from build123d import *

# Parameters (mm, degrees)
MODEL_R                  = 1.8
RESSALTO_EXTRUS_O1_DEPTH = 6


with BuildPart() as part:
    # Model → Ressalto-extrusão1 (new body)
    with BuildSketch(Plane.XY):
        Polygon((36.676362522, 11.559126959), (43.318311298, 11.559126959), (48.38117681, 16.621992471), (46.093165841, 35.592208395), (45.494331575, 40.442304919), (44.330954819, 41.605681674), (35.830954819, 41.605681674), (34.69889139, 40.473618245), (31.60820441, 16.627285071), align=None)
        with Locations((40.079692562, 35.592208395)):
            Circle(MODEL_R, mode=Mode.SUBTRACT)
    extrude(amount=RESSALTO_EXTRUS_O1_DEPTH)


solid = part.part
Read the model definition and answer for the solid it produces. Units are mm, in the model's axes. Coordinates: 2 decimals unless noted, no trailing zeros. Loops run counter-clockwise (first coordinate to the right, second up) from the corner with the lowest first, then second, coordinate; pieces in that order, holes last. Notation, with made-up numbers: (-3.75, 15.5) -> (8.25, 15.5) arc R26 ccw to (8.25, 40.5) -> close; hole circle Ø7 at (-12.5, 20.25). An arc over 180 degrees is marked (long way). Answer in a Markdown table with one row per item.
Item 1: A cutting plane is placed at B-B on x = 41.5. Determine the outline of the cut face in (y, z).
Returned:
| item | result |
|---|---|
| outline | (11.56, 0) -> (34.49, 0) -> (34.49, 6) -> (11.56, 6) -> close; (36.7, 0) -> (41.61, 0) -> (41.61, 6) -> (36.7, 6) -> close |
Item 2: This flat-tipped pin is pushed along its axis until it touches: P1, Ø4.5, axis at x = 40.08, y = 35.59, coming from the -Z side. Where does it stop, or does it pass through?
Returned:
| item | result |
|---|---|
| P1 | stops at z = 0 |
Item 3: A cutting plane is placed at A-A on z = 4.7. Determine the outline of the cut face in (x, y), plus the area to 3 significant figures.
Returned:
| item | result |
|---|---|
| outline | (31.61, 16.63) -> (36.68, 11.56) -> (43.32, 11.56) -> (48.38, 16.62) -> (46.09, 35.59) -> (45.49, 40.44) -> (44.33, 41.61) -> (35.83, 41.61) -> (34.7, 40.47) -> close; hole circle Ø3.6 at (40.08, 35.59) |
| area | 389 mm^2 |
Item 4: For a pull along X with two mould halves and no side action, classify faces 1 (the flat face through (35.273, 41.048, 2.958)), 2 (the flat face through (40, 41.606, 3)), 3 (the flat face through (44.921, 41.016, 2.958)), 4 (the cylindrical face through (41.797, 36.133, 2.958)) as released by +X, released by -X, zero draft, split by the parting line, or undercut.
Returned:
| item | result |
|---|---|
| face 1 | released by -X |
| face 2 | zero draft |
| face 3 | released by +X |
| face 4 | undercut |
Item 5: A cutting plane is placed at D-D on x = 34. Determine the outline of the cut face in (y, z), plus the area to 3 significant figures.
Returned:
| item | result |
|---|---|
| outline | (14.24, 0) -> (35.08, 0) -> (35.08, 6) -> (14.24, 6) -> close |
| area | 125 mm^2 |
Item 6: Straight lines are drawn through the part: line 1 along Y through (x, z) = (40.25, 0.7); line 2 along Y through (x, z) = (40.5, 3.45); line 3 along X through (y, z) = (18, 2). For each, find the intervals that lie inside material, in ascending order. Write a range as [from, to].
Returned:
| item | result |
|---|---|
| line 1 | y = [11.56, 33.8], [37.38, 41.61] |
| line 2 | y = [11.56, 33.84], [37.34, 41.61] |
| line 3 | x = [31.79, 48.21] |
Item 7: A cutting plane is placed at C-C on y = 37. Determine the outline of the cut face in (x, z), plus the area to 3 significant figures.
Returned:
| item | result |
|---|---|
| outline | (34.25, 0) -> (38.96, 0) -> (38.96, 6) -> (34.25, 6) -> close; (41.2, 0) -> (45.92, 0) -> (45.92, 6) -> (41.2, 6) -> close |
| area | 56.6 mm^2 |
